from build123d import *

# Parameters (mm, degrees)
F2_R     = 1.75
F3_DEPTH = 2
F4_R     = 14.5
F5_DEPTH = 5
F7_DEPTH = 12.9375
F8_SIZE  = 1.5


with BuildPart() as f1:
    # F0 (on Right) → F1 (revolve)
    with BuildSketch(Plane.YZ):
        with BuildLine():
            ThreePointArc((-11.1125, -6.7375), (-13.085868, -1.973368), (-17.85, 0))
            Line((-17.85, 0), (-17.85, -14))
            Line((-17.85, -14), (0, -14))
            Line((0, -14), (0, 0))
            ThreePointArc((0, 0), (-6.497722, -1.815933), (-11.1125, -6.7375))
        make_face()
    revolve(axis=Axis((0, 0, 9.125761), (0, 0, 1)))

    # F2 (on face) → F3 (join)
    with BuildSketch(Plane(origin=(0, 0, -14), x_dir=(1, 0, 0), z_dir=(0, 0, -1))):
        Polygon((-15.964466, -19.5), (0, -19.5), (15.964466, -19.5), (19.5, -15.964466), (19.5, 0), (19.5, 15.964466), (15.964466, 19.5), (0, 19.5), (-15.964466, 19.5), (-19.5, 15.964466), (-19.5, 0), (-19.5, -15.964466), align=None)
        with Locations((-15.202796, -15.202796)):
            Circle(F2_R, mode=Mode.SUBTRACT)
        with Locations((15.202796, -15.202796)):
            Circle(F2_R, mode=Mode.SUBTRACT)
        with Locations((-15.202796, 15.202796)):
            Circle(F2_R, mode=Mode.SUBTRACT)
        with Locations((15.202796, 15.202796)):
            Circle(F2_R, mode=Mode.SUBTRACT)
    extrude(amount=-F3_DEPTH)

    # F4 (on face) → F5 (join)
    with BuildSketch(Plane(origin=(0, 0, -14), x_dir=(1, 0, 0), z_dir=(0, 0, -1))):
        Circle(F4_R)
    extrude(amount=F5_DEPTH)

    # F6 (on face) → F7 (join)
    with BuildSketch(Plane(origin=(0, 0, -14), x_dir=(1, 0, 0), z_dir=(0, 0, -1))):
        Polygon((12.498112, 8.007984), (8.007984, 12.498112), (7.648774, 12.138902), (12.138902, 7.648774), align=None)
        Polygon((12.498112, -8.007984), (12.138902, -7.648774), (7.648774, -12.138902), (8.007984, -12.498112), align=None)
    extrude(amount=F7_DEPTH)

    # F8
    f8_edges = [f1.edges().sort_by_distance(p)[0] for p in [
        (12.318507, 7.828379, -26.9375),
        (7.828379, 12.318507, -26.9375),
        (7.828379, -12.318507, -26.9375),
        (12.318507, -7.828379, -26.9375),
    ]]
    chamfer(f8_edges, length=F8_SIZE)


solid = f1.part
Check sheet for the modelled part. Datum: model origin and axes. Units: mm. A direction names the side the tool comes from. Give positions to 0.01 mm unless a question says otherwise; leave off trailing zeros. Order: outer loops, then holes, each group sorted by start corner. A loop starts at its lowest first (then second) coordinate and runs counter-clockwise, first axis right, second up. Notation, with made-up numbers: M 5,60 L 19,60 A18 cw 19,75 Z; hole C -14.5,2 d10. An arc over 180 degrees is marked long. Answer as CSV lines item,"result". Start each with the question number.
Item 1: Thickness scan on line 1 (Z direction, x = 17, y = -13.5); line 2 (Z direction, x = 12, y = -13); line 3 (X direction, y = 3, z = -1.25). Record the ranges inside material, lowest first. Write a range as [from, to].
Item 2: Cross-section at D-D on z = -10.5. Enter the section's corners in (x, y), plus the area to 3 significant figures.
Item 3: Mould release check, pull along Y, two halves, no side actions. Record for faces 5 (the face through (-17.757, 17.707, -13.014)), 6 (the face through (16.87, -15.73, -13.01)), 7 (the face through (-19.5, 0, -13)): +Y half, -Y half, draft (parallel to the pull), parting line (faces both ways), or undercut.
Item 4: Cross-section at C-C on z = -5. State how many separate pieces and enclosed holes the cut face has, plus the area to 3 significant figures.
Item 5: Gauge pin test, flat ends, axial feed: P1, Ø2, axis at x = 0.5, y = -4, coming from the +Z side; P2, Ø4.5, axis at x = 15.2, y = 15.2, coming from the +Z side; P3, Ø4, axis at x = 4, z = -9.5, coming from the +Y side. Record the tip position at first contact, or that the pin passes through.
Item 6: Tool access check on faces 1 (the face through (9.93, 9.86, -22.91)), 2 (the face through (14.5, 0.1, -16.5)), 3 (the face through (10.222, 10.284, -20.378)), 4 (the face through (-14.494, -0.433, -16.465)). Record the directions out of +Z, -Z, +X, -X, +Y, -Y that give a thin tool (end or side, any length) a straight path to the whole face; none if there is none.
Item 7: Cross-section at A-A on z = -22.5. Enter the section's corners in (x, y).
Established:
1,line 1,"z = [-14, -12]"
1,line 2,"z = [-14, 0]"
1,line 3,"x = [-17.6, -13.61], [-4.56, 4.56], [13.61, 17.6]"
2,outline,"C 0,0 d35.7"
2,area,"1,000 mm^2"
3,face 5,"+Y half"
3,face 6,"undercut"
3,face 7,"draft"
4,separate pieces,"2"
4,enclosed holes,"1"
4,area,"912 mm^2"
5,P1,"stops at z = -0.37"
5,P2,"stops at z = -12"
5,P3,"stops at y = 17.74"
6,face 1,"-Z, -X"
6,face 2,"-Z, +X"
6,face 3,"-Z, +X, +Y"
6,face 4,"-Z"
7,outline,"M 7.65,-12.14 L 8.01,-12.5 L 12.5,-8.01 L 12.14,-7.65 Z; M 7.65,12.14 L 12.14,7.65 L 12.5,8.01 L 8.01,12.5 Z"
